Part model, mm, in its own coordinate system. Face numbers are marked on the shaded views. A direction names the side the tool comes from. Round coordinates to 2 decimals unless told otherwise and drop trailing zeros. Loops run counter-clockwise (first coordinate to the right, second up) from the corner with the lowest first, then second, coordinate; pieces in that order, holes last.
Autodesk Inventor part; units mm, degrees
ref_plane "YZ Plane" through (0, 0, 0) normal (1, 0, 0) x (0, 1, 0)
ref_plane "XZ Plane" through (0, 0, 0) normal (0, 1, 0) x (-1, 0, 0)
ref_plane "XY Plane" through (0, 0, 0) normal (0, 0, 1) x (1, 0, 0)
sketch "Эскиз1" plane through (0, 0, 0) normal (0, 1, 0) x (-1, 0, 0)
  circle A0 centre (0, 2.5) radius 0.75
  line L0 (0.9421, 0) -> (0.9421, 5)
  line L1 (0.9421, 5) -> (0, 5)
  arc A1 (0, 5) -> (0, 0) centre (0, 2.5) ccw
  line L2 (0.9421, 0) -> (0, 0)
  line L3 (0.9421, 0) -> (0.9421, 5)
  line L4 (6.9421, 0) -> (0.9421, 0)
  line L5 (6.9421, 5) -> (6.9421, 0)
  line L6 (0.9421, 5) -> (6.9421, 5)
  circle A2 centre (8, 2.5) radius 0.75
  line L7 (6.9421, 5) -> (6.9421, 0)
  line L8 (8, 0) -> (6.9421, 0)
  arc A3 (8, 0) -> (8, 5) centre (8, 2.5) ccw
  line L9 (8, 5) -> (6.9421, 5)
  line L10 (0.9421, 5) -> (6.9421, 5)
  line L11 (6.9421, 5) -> (6.9421, 4)
  line L12 (6.9421, 4) -> (0.9421, 4)
  line L13 (0.9421, 4) -> (0.9421, 5)
  point P0 (4, 5)
  dimension "d0" = 1
extrude "Выдавливание1" add sketch "Эскиз1" along normal blind 2 contours L2 A1 L1 L0 | L0 L12 L5 L4 | L5 L9 A3 L8
properties part number "КВ33.044.207 - Прижим ремня" material "Пластик АБС"
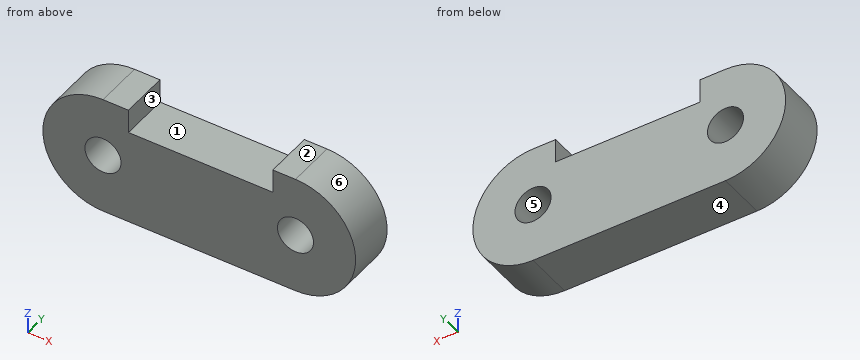
1) Slice it at B-B, the plane y = 1.3. Give the cut face in (x, z), then the cut area to 3 significant figures.
Values:
outline: (-8, 0) - (0, 0) arc R2.5 ccw to (0, 5) - (-0.94, 5) - (-0.94, 4) - (-6.94, 4) - (-6.94, 5) - (-8, 5) arc R2.5 ccw to start; hole circle Ø1.5 at (-8, 2.5); hole circle Ø1.5 at (0, 2.5)
area: 50.1 mm2
2) Drop flat-ended pins along their axis: pin 1 Ø0.5 at (y, z) = (0.5, 4.5) entering from -X; pin 2 Ø1 at (x, y) = (-3, 1) entering from +Z; pin 3 Ø0.5 at (y, z) = (1, 4.5) entering from +X. Give the stop position or say it passes through.
Values:
pin 1: stops at x = -9.79
pin 2: stops at z = 4
pin 3: stops at x = 1.79
3) Wall check: line 1 along Z through (x, y) = (-8, 0.45); line 2 along X through (y, z) = (1.15, 2.9); line 3 along Z through (x, y) = (-5, 1.6). Give the ranges that are in metal, low to high.
Values:
line 1: z = 0 to 1.75, 3.25 to 5
line 2: x = -10.47 to -8.63, -7.37 to -0.63, 0.63 to 2.47
line 3: z = 0 to 4
4) Slice it at A-A, the plane z = 2.5. Give the cut face in (x, y), then the cut area to 3 significant figures.
Values:
outline: (-10.5, 0) - (-8.75, 0) - (-8.75, 2) - (-10.5, 2) - close; (-7.25, 0) - (-0.75, 0) - (-0.75, 2) - (-7.25, 2) - close; (0.75, 0) - (2.5, 0) - (2.5, 2) - (0.75, 2) - close
area: 20.0 mm2
5) Slice it at D-D, the plane z = 4.45. Give the cut face in (x, y), then the cut area to 3 significant figures.
Values:
outline: (-9.56, 0) - (-6.94, 0) - (-6.94, 2) - (-9.56, 2) - close; (-0.94, 0) - (1.56, 0) - (1.56, 2) - (-0.94, 2) - close
area: 10.3 mm2
6) Tool access for the marked faces 1 and 2: list every direction of +Z, -Z, +X, -X, +Y, -Y with a clear straight run to the whole face (end or side of a thin tool).
Values:
face 1: +Z, +Y, -Y
face 2: +Z, +X, -X, +Y, -Y
7) Mould opens along X. For the marked faces 3, 4, 5 and 6 say: released by +X, released by -X, zero draft, split by the parting line, or undercut.
Values:
face 3: undercut
face 4: zero draft
face 5: undercut
face 6: released by +X
8) Slice it at C-C, the plane x = 0.5. Give the cut face in (y, z).
Values:
outline: (0, 0.05) - (2, 0.05) - (2, 1.94) - (0, 1.94) - close; (0, 3.06) - (2, 3.06) - (2, 4.95) - (0, 4.95) - close
